Here's how the part is built. I have some questions about the finished solid (model axes, mm). A direction names the side the tool comes from. Round coordinates to 2 decimals unless told otherwise and drop trailing zeros. Use one line per item in the form item = value. Start each with the question number.
Item 1: If I drill on L1, parallel to Y at x = 8.5, z = 0.75; L2, parallel to Y at x = -8.5, z = 4.5; L3, parallel to Y at x = -6.5, z = 4, over which ranges is the centre line in solid material (lowest first)? Write a range as [from, to].
Item 2: I'm going to push flat-ended pins straight in: pin 1 Ø2 at (x, z) = (8.5, 13) entering from +Y; pin 2 Ø2 at (x, z) = (-41, 1.5) entering from +Y; pin 3 Ø6 at (x, y) = (28.5, -3) entering from +Z; pin 4 Ø4 at (x, z) = (-2, 4) entering from +Y. Where does each tip first touch, or does it pass through?
Item 3: For faces 1 (the face through (-2.765, -23.577, 0.76)), 2 (the face through (-1.575, -41.087, -1.232)), 3 (the face through (-19.404, 3.293, 2.26)), which set-ups out of +Z, -Z, +X, -X, +Y, -Y let a thin tool reach every point of the face, with its end or its side?
Item 4: Thinking about a two-plate mould opening in X: for faces 4 (the face through (1, 39, -2.5)), 5 (the face through (-12.376, -41.575, 1.479)), 6 (the face through (-11.28, -20.11, 0.76)), which applies, released by +X, released by -X, zero draft, split by the parting line, or undercut?
```python
from build123d import *

# Parameters (mm, degrees)
F1_ANGLE  = 180
F2_R      = 11
F3_DEPTH  = 3.5
F4_R      = 10.5
F5_DEPTH  = 25
F6_R      = 17.5
F7_DEPTH  = 3
F8_R      = 2.84
F9_DEPTH  = 1.5
F10_R     = 1.5
F11_DEPTH = 25
F12_R     = 2
F13_DEPTH = 2.5


with BuildPart() as f1:
    # F0 (on Top) → F1 (revolve)
    with BuildSketch(Plane.XY):
        with BuildLine():
            ThreePointArc((0, -18.5), (13.081475, -13.081475), (18.5, 0))
            ThreePointArc((18.5, 0), (13.081475, 13.081475), (0, 18.5))
            Line((0, 18.5), (0, -18.5))
        make_face()
    revolve(axis=Axis((0, 0, 0), (0, -1, 0)), revolution_arc=F1_ANGLE)

    # F2 (on face) → F3 (cut)
    with BuildSketch(Plane(origin=(0, 0, 0), x_dir=(1, 0, 0), z_dir=(0, 0, -1))):
        Circle(F2_R)
    extrude(amount=-F3_DEPTH, mode=Mode.SUBTRACT)

    # F4 (on face) → F5 (cut)
    with BuildSketch(Plane(origin=(0, 0, 3.5), x_dir=(1, 0, 0), z_dir=(0, 0, -1))):
        Circle(F4_R)
    extrude(amount=-F5_DEPTH, mode=Mode.SUBTRACT)

    # F6 (on face) → F7 (join)
    with BuildSketch(Plane(origin=(0, 0, 0), x_dir=(1, 0, 0), z_dir=(0, 0, -1))):
        with BuildLine():
            ThreePointArc((13.435029, 13.435029), (2.776181, 37.480821), (3.703777, 63.766763))
            ThreePointArc((3.703777, 63.766763), (-12.505008, 41.202234), (-13.435029, 13.435029))
            ThreePointArc((-13.435029, 13.435029), (-37.480821, 2.776181), (-63.766763, 3.703777))
            ThreePointArc((-63.766763, 3.703777), (-41.202234, -12.505008), (-13.435029, -13.435029))
            ThreePointArc((-13.435029, -13.435029), (-2.776181, -37.480821), (-3.703777, -63.766763))
            ThreePointArc((-3.703777, -63.766763), (12.505008, -41.202234), (13.435029, -13.435029))
            ThreePointArc((13.435029, -13.435029), (37.480821, -2.776181), (63.766763, -3.703777))
            ThreePointArc((63.766763, -3.703777), (41.202234, 12.505008), (13.435029, 13.435029))
        make_face()
        Circle(F6_R, mode=Mode.SUBTRACT)
    extrude(amount=-F7_DEPTH)

    # F8 (on face) → F9 (cut)
    with BuildSketch(Plane.XY.offset(3)):
        with Locations((-11.08485, -21.599201)):
            Circle(F8_R)
        with Locations((-2.440276, -22.113062)):
            Circle(F8_R)
        with Locations((-10.892785, -28.53697)):
            Circle(F8_R)
        with Locations((-3.961728, -28.87507)):
            Circle(F8_R)
        with Locations((-7.655934, -35.751011)):
            Circle(F8_R)
        with Locations((-6.942718, -43.498125)):
            Circle(F8_R)
        with Locations((-2.119637, -51.609669)):
            Circle(F8_R)
        with Locations((21.599201, -11.08485)):
            Circle(F8_R)
        with Locations((22.113062, -2.440276)):
            Circle(F8_R)
        with Locations((28.53697, -10.892785)):
            Circle(F8_R)
        with Locations((28.87507, -3.961728)):
            Circle(F8_R)
        with Locations((35.751011, -7.655934)):
            Circle(F8_R)
        with Locations((43.498125, -6.942718)):
            Circle(F8_R)
        with Locations((51.609669, -2.119637)):
            Circle(F8_R)
        with Locations((11.08485, 21.599201)):
            Circle(F8_R)
        with Locations((2.440276, 22.113062)):
            Circle(F8_R)
        with Locations((10.892785, 28.53697)):
            Circle(F8_R)
        with Locations((3.961728, 28.87507)):
            Circle(F8_R)
        with Locations((7.655934, 35.751011)):
            Circle(F8_R)
        with Locations((6.942718, 43.498125)):
            Circle(F8_R)
        with Locations((2.119637, 51.609669)):
            Circle(F8_R)
        with Locations((-21.599201, 11.08485)):
            Circle(F8_R)
        with Locations((-22.113062, 2.440276)):
            Circle(F8_R)
        with Locations((-28.53697, 10.892785)):
            Circle(F8_R)
        with Locations((-28.87507, 3.961728)):
            Circle(F8_R)
        with Locations((-35.751011, 7.655934)):
            Circle(F8_R)
        with Locations((-43.498125, 6.942718)):
            Circle(F8_R)
        with Locations((-51.609669, 2.119637)):
            Circle(F8_R)
    extrude(amount=-F9_DEPTH, mode=Mode.SUBTRACT)

    # F10 (on face) → F11 (cut)
    with BuildSketch(Plane.XY.offset(3)):
        with Locations((-2.440276, -22.113062)):
            Circle(F10_R)
        with Locations((-22.113062, 2.440276)):
            Circle(F10_R)
        with Locations((2.440276, 22.113062)):
            Circle(F10_R)
        with Locations((22.113062, -2.440276)):
            Circle(F10_R)
        with Locations((-11.08485, -21.599201)):
            Circle(F10_R)
        with Locations((-10.892785, -28.53697)):
            Circle(F10_R)
        with Locations((-3.961728, -28.87507)):
            Circle(F10_R)
        with Locations((-7.655934, -35.751011)):
            Circle(F10_R)
        with Locations((-6.942718, -43.498125)):
            Circle(F10_R)
        with Locations((-2.119637, -51.609669)):
            Circle(F10_R)
        with Locations((21.599201, -11.08485)):
            Circle(F10_R)
        with Locations((28.53697, -10.892785)):
            Circle(F10_R)
        with Locations((28.87507, -3.961728)):
            Circle(F10_R)
        with Locations((35.751011, -7.655934)):
            Circle(F10_R)
        with Locations((43.498125, -6.942718)):
            Circle(F10_R)
        with Locations((51.609669, -2.119637)):
            Circle(F10_R)
        with Locations((11.08485, 21.599201)):
            Circle(F10_R)
        with Locations((10.892785, 28.53697)):
            Circle(F10_R)
        with Locations((3.961728, 28.87507)):
            Circle(F10_R)
        with Locations((7.655934, 35.751011)):
            Circle(F10_R)
        with Locations((6.942718, 43.498125)):
            Circle(F10_R)
        with Locations((2.119637, 51.609669)):
            Circle(F10_R)
        with Locations((-21.599201, 11.08485)):
            Circle(F10_R)
        with Locations((-28.53697, 10.892785)):
            Circle(F10_R)
        with Locations((-28.87507, 3.961728)):
            Circle(F10_R)
        with Locations((-35.751011, 7.655934)):
            Circle(F10_R)
        with Locations((-43.498125, 6.942718)):
            Circle(F10_R)
        with Locations((-51.609669, 2.119637)):
            Circle(F10_R)
    extrude(amount=-F11_DEPTH, mode=Mode.SUBTRACT)

    # F12 (on face) → F13 (join)
    with BuildSketch(Plane(origin=(0, 0, 0), x_dir=(1, 0, 0), z_dir=(0, 0, -1))):
        with Locations((-23.183173, 3.233931)):
            Circle(F12_R)
        with Locations((-39.104387, -1.314987)):
            Circle(F12_R)
        with Locations((-3.233931, -23.183173)):
            Circle(F12_R)
        with Locations((1.314987, -39.104387)):
            Circle(F12_R)
        with Locations((23.183173, -3.233931)):
            Circle(F12_R)
        with Locations((39.104387, 1.314987)):
            Circle(F12_R)
        with Locations((3.233931, 23.183173)):
            Circle(F12_R)
        with Locations((-1.314987, 39.104387)):
            Circle(F12_R)
    extrude(amount=F13_DEPTH)


solid = f1.part
```
Values found:
q1.L1 = [-21.22, -6.98], [6.98, 34.51], [36.99, 49.96]
q1.L2 = [-15.8, -6.16], [6.16, 15.8]
q1.L3 = [-16.85, -8.25], [8.25, 16.85]
q2.pin_1 = 11.45
q2.pin_2 = 12.9
q2.pin_3 = 3
q2.pin_4 = 63.77
q3.face_1 = +Z, -Z
q3.face_2 = -Z
q3.face_3 = +Z
q4.face_4 = zero draft
q4.face_5 = released by -X
q4.face_6 = undercut
